Source: CAD feature listing. Evaluate the final solid. Frame: model axes, mm. A direction names the side the tool comes from. Coordinates: 2 decimals unless noted, no trailing zeros. Order: outer loops, then holes, each group sorted by start corner. A loop starts at its lowest first (then second) coordinate and runs counter-clockwise, first axis right, second up. Notation, with made-up numbers: (19.25, -3) -> (54.25, -3) arc R21 ccw to (54.25, 10) -> close; hole circle Ø2 at (89, -9). An arc over 180 degrees is marked (long way). Write item = value, one per line. Start each with the question number.
Item 1: Contact query for flat-ended pins moving along their axis: pin 1 (5 mm diameter, centred on y = -7, z = 4.5, fed in from +X); pin 2 (1.5 mm diameter, centred on x = 1.5, z = 0, fed in from -Y); pin 3 (2 mm diameter, centred on x = 6.5, y = -6.5, fed in from +Z); pin 4 (13.5 mm diameter, centred on x = -2, z = 0, fed in from -Y). Output: stop coordinate, or through.
Item 2: Section query B-B (y = 1.5). Output: boundary loops of the cut face in (x, z), then the cut area to 3 significant figures.
Item 3: Section query A-A (x = -2). Output: boundary loops of the cut face in (y, z).
Item 4: Mould query, pull axis Z, two halves, no side actions, for faces 1 (the conical face through (-7.09, -10.9, 10.07)), 2 (the flat face through (3, -15.5, 2)), 3 (the flat face through (0, 0, -16)). Classes: released by +Z, released by -Z, zero draft, split by the parting line, or undercut.
Item 5: Set-up query: faces 4 (the flat face through (4.3, -10.9, -8.3)), 5 (the flat face through (-1.99, -10.9, -10.31)), 6 (the flat face through (14, -3.5, -0.2)), 7 (the flat face through (-13, -4, -7)), 8 (the flat face through (6, 3, -4)). Return all of +Z, -Z, +X, -X, +Y, -Y with unobstructed straight access to the full face (end or side cutting, diameter ignored); none if empty.
Item 6: Section query C-C (z = 0). Output: boundary loops of the cut face in (x, y).
Item 7: Ray query, line 1 along X through (y, z) = (-3.25, 0); line 2 along Y through (x, z) = (-4.5, -11.5); line 3 along Z through (x, y) = (-2, -16.6). Return the intervals inside material, ascending. Write a range as [from, to].
Autodesk Inventor part; units mm, degrees
ref_plane "insrt_to_lock_XY" through (-2, 3, 0) normal (0, 1, 0) x (1, 0, 0)
ref_plane "insrt_to_lock_YZ" through (-2, 3, 0) normal (1, 0, 0) x (0, 0, -1)
ref_plane "insrt_to_lock_ZX" through (-2, 3, 0) normal (0, 0, -1) x (0, 1, 0)
sketch "Sketch_1" plane through (0, 0, 0) normal (0, 0, 1) x (1, 0, 0)
  line L0 (-18, -4) -> (14, -4)
  line L1 (14, -4) -> (14, -3)
  line L2 (14, -3) -> (18, 1)
  line L3 (18, 1) -> (18, 3)
  line L4 (18, 3) -> (-14, 3)
  line L5 (-14, 3) -> (-18, -1)
  line L6 (-18, -1) -> (-18, -4)
extrude "Extrusion1" add sketch "Sketch_1" along normal mid plane 32
sketch "Sketch_2" plane through (0, -3, 0) normal (0, 1, 0) x (1, 0, 0)
  arc A0 (-13.055, -4.46) -> (-11.555, -5.96) centre (-11.555, -4.46) ccw
  line L0 (-11.555, -5.96) -> (-11.045, -5.96)
  line L1 (-11.045, -5.96) -> (-11.045, -7.49)
  arc A1 (-11.045, -7.49) -> (-9.545, -8.99) centre (-9.545, -7.49) ccw
  line L2 (-9.545, -8.99) -> (-8.015, -8.99)
  line L3 (-8.015, -8.99) -> (-8.015, -9.5)
  arc A2 (-8.015, -9.5) -> (-6.515, -11) centre (-6.515, -9.5) ccw
  line L4 (-6.515, -11) -> (2.405, -11)
  arc A3 (2.405, -11) -> (3.905, -9.5) centre (2.405, -9.5) ccw
  line L5 (3.905, -9.5) -> (3.905, -8.99)
  line L6 (3.905, -8.99) -> (5.435, -8.99)
  arc A4 (5.435, -8.99) -> (6.935, -7.49) centre (5.435, -7.49) ccw
  line L7 (6.935, -7.49) -> (6.935, -5.96)
  line L8 (6.935, -5.96) -> (7.445, -5.96)
  arc A5 (7.445, -5.96) -> (8.945, -4.46) centre (7.445, -4.46) ccw
  line L9 (8.945, -4.46) -> (8.945, 4.46)
  arc A6 (8.945, 4.46) -> (7.445, 5.96) centre (7.445, 4.46) ccw
  line L10 (7.445, 5.96) -> (6.935, 5.96)
  line L11 (6.935, 5.96) -> (6.935, 7.49)
  arc A7 (6.935, 7.49) -> (5.435, 8.99) centre (5.435, 7.49) ccw
  line L12 (5.435, 8.99) -> (3.905, 8.99)
  line L13 (3.905, 8.99) -> (3.905, 9.5)
  arc A8 (3.905, 9.5) -> (2.405, 11) centre (2.405, 9.5) ccw
  line L14 (2.405, 11) -> (-6.515, 11)
  arc A9 (-6.515, 11) -> (-8.015, 9.5) centre (-6.515, 9.5) ccw
  line L15 (-8.015, 9.5) -> (-8.015, 8.99)
  line L16 (-8.015, 8.99) -> (-9.545, 8.99)
  arc A10 (-9.545, 8.99) -> (-11.045, 7.49) centre (-9.545, 7.49) ccw
  line L17 (-11.045, 7.49) -> (-11.045, 5.96)
  line L18 (-11.045, 5.96) -> (-11.555, 5.96)
  arc A11 (-11.555, 5.96) -> (-13.055, 4.46) centre (-11.555, 4.46) ccw
  line L19 (-13.055, 4.46) -> (-13.055, -4.46)
extrude "Extrusion2" add sketch "Sketch_2" against normal blind 15 draft -5
sketch "Sketch3" plane through (-14, 3, 16) normal (0, 1, 0) x (1, 0, 0)
  point P0 (12, 16)
hole "Hole1" at (-2, 3, 0) direction (0, -1, 0) diameter 10.2 depth 21 counterbore diameter 16 counterbore depth 18.5
ref_plane "insrt_to_lock_XY" through (-2, 3, 0) normal (0, 1, 0) x (1, 0, 0)
ref_plane "insrt_to_lock_YZ" through (-2, 3, 0) normal (1, 0, 0) x (0, 0, -1)
ref_plane "insrt_to_lock_ZX" through (-2, 3, 0) normal (0, 0, -1) x (0, 1, 0)
ref_plane "lock_to_body_XY" through (0, 3, 0) normal (0, 1, 0) x (1, 0, 0)
ref_plane "lock_to_body_YZ" through (0, 3, 0) normal (1, 0, 0) x (0, 0, -1)
ref_plane "lock_to_body_ZX" through (0, 3, 0) normal (0, 0, -1) x (0, 1, 0)
ref_plane "washer_XY" through (-2, -18.5, 0) normal (0, 1, 0) x (1, 0, 0)
ref_plane "washer_YZ" through (-2, -18.5, 0) normal (1, 0, 0) x (0, 0, -1)
ref_plane "washer_ZX" through (-2, -18.5, 0) normal (0, 0, -1) x (0, 1, 0)
properties part number "wm_one_door_lock_na"
Computed:
q1.pin_1 = 8.81
q1.pin_2 = through
q1.pin_3 = 8.71
q1.pin_4 = -18
q2.outline = (-15.5, -16) -> (18, -16) -> (18, 16) -> (-15.5, 16) -> close; hole circle Ø16 at (-2, 0)
q2.area = 871 mm^2
q3.outline = (-18, -9.69) -> (-4, -10.91) -> (-4, -16) -> (3, -16) -> (3, -8) -> (-15.5, -8) -> (-15.5, -5.1) -> (-18, -5.1) -> close; (-18, 5.1) -> (-15.5, 5.1) -> (-15.5, 8) -> (3, 8) -> (3, 16) -> (-4, 16) -> (-4, 10.91) -> (-18, 9.69) -> close
q4.face_1 = released by +Z
q4.face_2 = undercut
q4.face_3 = released by -Z
q5.face_4 = -Z, +X, -Y
q5.face_5 = -Z, +X, -X, -Y
q5.face_6 = +Z, -Z, +X, -Y
q5.face_7 = -Y
q5.face_8 = +Z, -Z, +X, -X, +Y
q6.outline = (-18, -4) -> (-12.97, -4) -> (-11.74, -18) -> (-7.1, -18) -> (-7.1, -15.5) -> (-10, -15.5) -> (-10, 3) -> (-14, 3) -> (-18, -1) -> close; (3.1, -18) -> (7.63, -18) -> (8.86, -4) -> (14, -4) -> (14, -3) -> (18, 1) -> (18, 3) -> (6, 3) -> (6, -15.5) -> (3.1, -15.5) -> close
q7.line_1 = [-18, -10], [6, 14]
q7.line_2 = [-4, 3]
q7.line_3 = [-9.81, -5.1], [5.1, 9.81]
